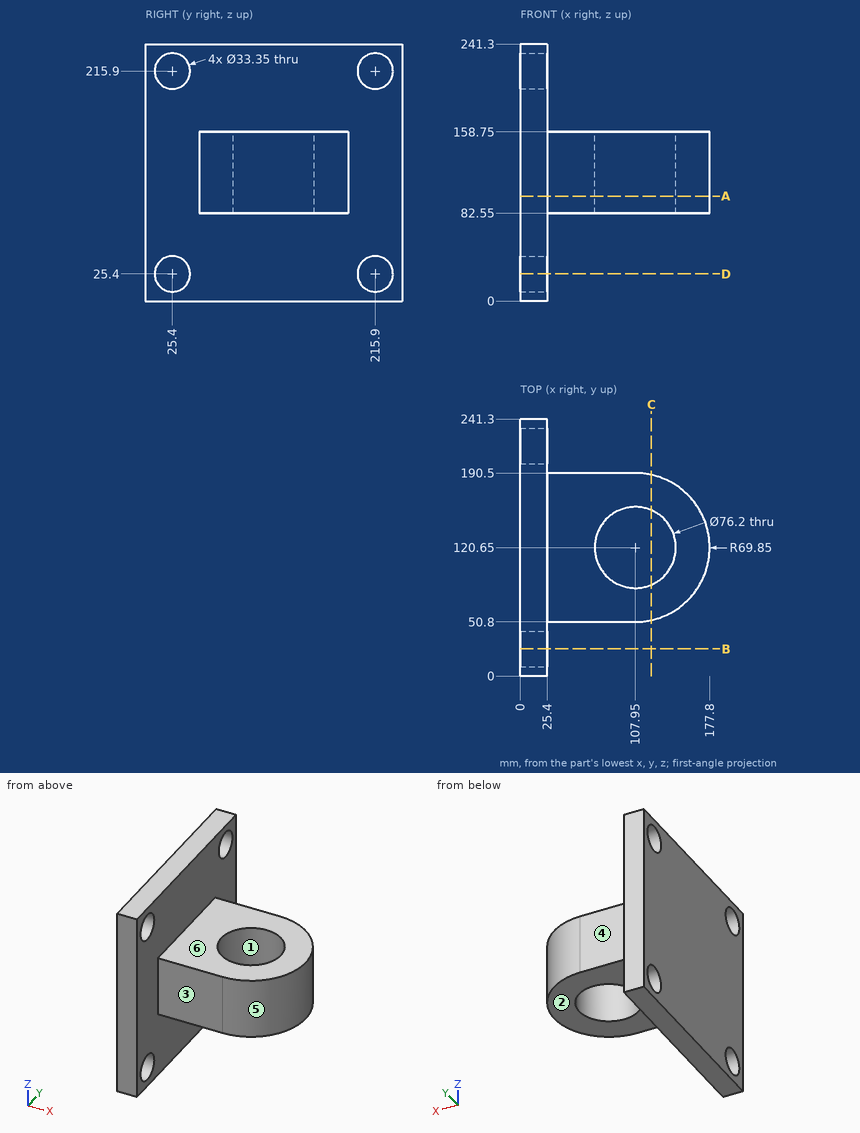
The figure shows three views and two pictorial views of one solid part (mm, origin at its lowest corner). Answer the questions. A direction names the side the tool comes from. Round coordinates to 2 decimals unless told otherwise and drop trailing zeros. Order: outer loops, then holes, each group sorted by start corner. A loop starts at its lowest first (then second) coordinate and runs counter-clockwise, first axis right, second up. Notation, with made-up numbers: M 43.5,76 L 74.5,76 A25 ccw 74.5,95 Z; hole C 63.5,17.5 d6. An arc over 180 degrees is marked long. Answer in a Markdown table with one row per item. Add a question column.
1) Consider line 1 along Y through (x, z) = (12.25, 25.4) (1 decimal); line 2 along Y through (x, z) = (6, 215); line 3 along X through (y, z) = (150.5, 206.5). Determine where each line is inside the solid, lowest interval first. Write a range as from..to.
2) Which of the six approach directions +Z, -Z, +X, -X, +Y, -Y give full straight-line access (tool end or side, diameter ignored) to the marked faces 4, 5 and 6?
3) The part is cut by section C-C on x = 123. Determine the outline of the cut face in (y, z), plus the area to 3 significant figures.
4) Determine the mould class of the marked faces 1, 2 and 3 for opening direction Y: pulls with the +Y half, pulls with the -Y half, needs draft (parallel to the pull), parting line crosses it, or undercut.
5) The part is cut by section A-A on z = 98.5. Determine the outline of the cut face in (x, y), plus the area to 3 significant figures.
6) The part is cut by section B-B on y = 25.4. Determine the outline of the cut face in (x, z) (1 decimal), plus the area to 4 significant figures.
7) Flat-ended cylindrical pins translate along their axes: pin 1 Ø4 at (y, z) = (69, 137.5) entering from +X; pin 2 Ø3 at (y, z) = (63.5, 43.5) entering from +X. Find the tip coordinate at first contact, or state that the pin passes through.
Findings below:
| question | item | result |
|---|---|---|
| 1 | line 1 | y = 0..8.7, 42.1..199.2, 232.6..241.3 |
| 1 | line 2 | y = 0..8.75, 42.05..199.25, 232.55..241.3 |
| 1 | line 3 | x = 0..25.4 |
| 2 | face 4 | +Z, -Z, +X, +Y |
| 2 | face 5 | +Z, -Z, +X |
| 2 | face 6 | +Z, +X, +Y, -Y |
| 3 | outline | M 52.44,82.55 L 85.65,82.55 L 85.65,158.75 L 52.44,158.75 Z; M 155.65,82.55 L 188.86,82.55 L 188.86,158.75 L 155.65,158.75 Z |
| 3 | area | 5,060 mm² |
| 4 | face 1 | undercut |
| 4 | face 2 | needs draft |
| 4 | face 3 | pulls with the -Y half |
| 5 | outline | M 0,0 L 25.4,0 L 25.4,50.8 L 107.95,50.8 A69.85 ccw 107.95,190.5 L 25.4,190.5 L 25.4,241.3 L 0,241.3 Z; hole C 107.95,120.65 d76.2 |
| 5 | area | 20,800 mm² |
| 6 | outline | M 0,0 L 25.4,0 L 25.4,8.7 L 0,8.7 Z; M 0,42.1 L 25.4,42.1 L 25.4,199.2 L 0,199.2 Z; M 0,232.6 L 25.4,232.6 L 25.4,241.3 L 0,241.3 Z |
| 6 | area | 4,435 mm² |
| 7 | pin 1 | stops at x = 157.08 |
| 7 | pin 2 | stops at x = 25.4 |
